The model under review builds one solid part; all positions refer to its coordinate system, in mm. A direction names the side the tool comes from. Give positions to 0.01 mm unless a question says otherwise; leave off trailing zeros. Loops run counter-clockwise (first coordinate to the right, second up) from the corner with the lowest first, then second, coordinate; pieces in that order, holes last. Notation, with made-up numbers: (76, -1) -> (131, -1) arc R10 cw to (131, 18) -> close; hole circle Ø9 at (34, 1). An arc over 180 degrees is marked (long way). Write each question's results on one line, items separated by ' | '. Start each with the question number.
Q1. We need section A-A (z = -9). Write out the cut boundary in (x, y).
Q2. Mouldability with a two-part tool opening along X and no side actions: class faces 1 (the face through (-13.6, 6.26, -7.86)), 2 (the face through (-13.79, 5.01, 1.7)), 3 (the face through (-22, 12.7, -6)) as released by +X, released by -X, zero draft, split by the parting line, or undercut.
Q3. Machinability: for faces 4 (the face through (-17, 0, -5)), 5 (the face through (-17, 10.16, 3)), which of the approach directions +Z, -Z, +X, -X, +Y, -Y give a long, thin tool a straight path to every point of the face, cutting with its end or side? Answer none if there is none.
Q4. We need section D-D (y = 11.5). Write out the cut boundary in (x, z), plus the area to 3 significant figures.
Q5. Wall thickness on L1, parallel to Z at x = -20.5, y = 12; L2, parallel to X at y = 4.25, z = -12.5; L3, parallel to X at y = 4.5, z = -10.5: over which ranges is each line inside the solid? List them lowest first. Write a range as [from, to].
Q6. Insertion check: pin 1 Ø1.5 at (y, z) = (2.5, 3.5) entering from -X; pin 2 Ø1.5 at (x, z) = (-3, -13) entering from -Y; pin 3 Ø1 at (y, z) = (3, 0.5) entering from -X; pin 4 Ø4 at (y, z) = (2, -11) entering from +X. Each pin has a flat end and moves straight along its axis. Give the tip position at first contact, or say it passes through.
Q7. We need section C-C (z = -22). Write out the cut boundary in (x, y).
Q8. We need section B-B (x = -11). Write out the cut boundary in (y, z).
from build123d import *

# Parameters (mm, degrees)
SKETCH1_R           = 12.7
BOSS_EXTRUDE1_DEPTH = 10.16
SKETCH2_R           = 19.84375
SKETCH2_R_2         = 4.7498
BOSS_EXTRUDE2_DEPTH = 2.54
CUT_EXTRUDE1_START  = -12.7
SKETCH3_R           = 4.7498
CUT_EXTRUDE1_DEPTH  = 12.7


with BuildPart() as part:
    # Sketch1 → Boss-Extrude1 (new body)
    with BuildSketch(Plane(origin=(0, 0, 0), x_dir=(1, 0, 0), z_dir=(0, 1, 0))):
        with Locations(Location((-17.607350735, 10.410900498, 0), (0, 0, 270))):
            Circle(SKETCH1_R)
    extrude(amount=BOSS_EXTRUDE1_DEPTH)

    # Sketch2 → Boss-Extrude2 (add)
    with BuildSketch(Plane(origin=(0, 10.16, 0), x_dir=(1, 0, 0), z_dir=(0, 1, 0))):
        with Locations(Location((-17.607350735, 10.410900498, 0), (0, 0, 270))):
            Circle(SKETCH2_R)
        with Locations(Location((-17.607350735, 10.410900498, 0), (0, 0, 270))):
            Circle(SKETCH2_R_2, mode=Mode.SUBTRACT)
    extrude(amount=BOSS_EXTRUDE2_DEPTH)

    # Sketch3 → Cut-Extrude1 (cut)
    with BuildSketch(Plane(origin=(0, 10.16, 0), x_dir=(1, 0, 0), z_dir=(0, 1, 0)).offset(CUT_EXTRUDE1_START)):
        with Locations(Location((-17.607350735, 10.410900498, 0), (0, 0, 270))):
            Circle(SKETCH3_R)
    extrude(amount=CUT_EXTRUDE1_DEPTH, mode=Mode.SUBTRACT)


solid = part.part
Output:
1) outline: (-37.4, 10.16) -> (-30.23, 10.16) -> (-30.23, 0) -> (-22.14, 0) -> (-22.14, 12.7) -> (-37.4, 12.7) -> close; (-13.07, 0) -> (-4.99, 0) -> (-4.99, 10.16) -> (2.19, 10.16) -> (2.19, 12.7) -> (-13.07, 12.7) -> close
2) face 1: undercut | face 2: split by the parting line | face 3: zero draft
3) face 4: +Z, -Z, +X, -X, -Y | face 5: -Y
4) outline: circle Ø39.69 at (-17.61, -10.41); hole circle Ø9.5 at (-17.61, -10.41) | area: 1,170 mm2
5) L1: [-30.04, -14.18], [-6.64, 9.22] | L2: [-30.13, -21.87], [-13.34, -5.08] | L3: [-30.31, -22.36], [-12.86, -4.91]
6) pin 1: through | pin 2: y = 10.16 | pin 3: x = -24.88 | pin 4: x = -4.91
7) outline: (-33.72, 10.16) -> (-22.8, 10.16) -> (-22.8, 0) -> (-12.41, 0) -> (-12.41, 10.16) -> (-1.5, 10.16) -> (-1.5, 12.7) -> (-33.72, 12.7) -> close
8) outline: (0, -21.26) -> (10.16, -21.26) -> (10.16, -29.12) -> (12.7, -29.12) -> (12.7, 8.3) -> (10.16, 8.3) -> (10.16, 0.43) -> (0, 0.43) -> close
